Design review of the part built by this model. Coordinates are the model's own, in mm. Face numbers are marked on the shaded views. Coordinates: 2 decimals unless noted, no trailing zeros. Write each loop counter-clockwise with the first axis right and the second up, starting at its lowest first coordinate (ties: lowest second). Pieces come first, ordered by that corner, then holes.
Q1. To check wall thickness, follow probe 1 along Y at (x, z) = (0, -5.75); probe 2 along X at (y, z) = (5, -10.5); probe 3 along X at (y, z) = (-34.5, -4.25). State the ranges of each line that lie inside material, in increasing order.
Q2. Add section A-A, the plane x = 0. Give the boundary of the cut face in (y, z).
Q3. Clearance check with flat-ended pins moving along their axes: pin 1 Ø10 at (y, z) = (-42, -6) entering from -X; pin 2 Ø1.5 at (y, z) = (62, 1.5) entering from -X; pin 3 Ø10 at (x, z) = (4, -1) entering from +Y. State where each tip first meets the part, or that it passes through.
Q4. Add section B-B, the plane z = -6.5. Give the boundary of the cut face in (x, y), plus the area to 3 significant figures.
Q5. The part is to be moulded in two halves that separate along X. For the marked faces 1, 2, 3 and 4, say which applies: +X half, -X half, draft (parallel to the pull), parting line (faces both ways), or undercut.
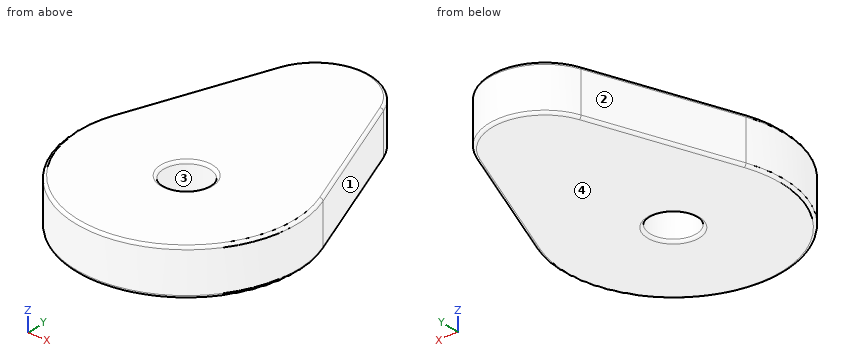
from build123d import *

# Parameters (mm, degrees)
SKETCH1_R           = 12.5
BOSS_EXTRUDE1_DEPTH = 12.5
FILLET1_R           = 1.5
FILLET2_R           = 1.5


with BuildPart() as part:
    # Sketch1 → Boss-Extrude1 (new, symmetric)
    with BuildSketch(Plane.XY):
        with BuildLine():
            Line((-56.159743046, 21.120683252), (-28.079871523, 95.784857261))
            ThreePointArc((-28.079871523, 95.784857261), (0, 115.224515635), (28.079871523, 95.784857261))
            Line((28.079871523, 95.784857261), (56.159743046, 21.120683252))
            ThreePointArc((56.159743046, 21.120683252), (0, -60), (-56.159743046, 21.120683252))
        make_face()
        Circle(SKETCH1_R, mode=Mode.SUBTRACT)
    extrude(amount=BOSS_EXTRUDE1_DEPTH, both=True)

    # Fillet1
    fillet1_edges = [part.edges().sort_by_distance(p)[0] for p in [
        (0, 115.224515635, 12.5),
        (-42.119807284, 58.452770256, 12.5),
        (0, -60, 12.5),
        (-42.119807284, 58.452770256, -12.5),
        (0, 115.224515635, -12.5),
        (42.119807284, 58.452770256, -12.5),
        (0, -60, -12.5),
        (42.119807284, 58.452770256, 12.5),
    ]]
    fillet(fillet1_edges, radius=FILLET1_R)

    # Fillet2
    fillet2_edges = [part.edges().sort_by_distance(p)[0] for p in [
        (-12.5, 0, -12.5),
        (-12.5, 0, 12.5),
    ]]
    fillet(fillet2_edges, radius=FILLET2_R)


solid = part.part
Here are the results:
1. probe 1: y = -60 to -12.5, 12.5 to 115.22
1. probe 2: x = -59.79 to -11.46, 11.46 to 59.79
1. probe 3: x = -49.09 to 49.09
2. outline: (-60, -11) arc R1.5 ccw to (-58.5, -12.5) - (-14, -12.5) arc R1.5 ccw to (-12.5, -11) - (-12.5, 11) arc R1.5 ccw to (-14, 12.5) - (-58.5, 12.5) arc R1.5 ccw to (-60, 11) - close; (12.5, -11) arc R1.5 ccw to (14, -12.5) - (113.72, -12.5) arc R1.5 ccw to (115.22, -11) - (115.22, 11) arc R1.5 ccw to (113.72, 12.5) - (14, 12.5) arc R1.5 ccw to (12.5, 11) - close
3. pin 1: stops at x = -47.23
3. pin 2: stops at x = -41.07
3. pin 3: stops at y = 115.22
4. outline: (-56.16, 21.12) arc R60 ccw (long way) to (56.16, 21.12) - (28.08, 95.78) arc R30 ccw to (-28.08, 95.78) - close; hole circle Ø25 at (0, 0)
4. area: 14,700 mm2
5. face 1: +X half
5. face 2: -X half
5. face 3: undercut
5. face 4: draft
